The listing builds one solid part. Answer for the finished solid, in the listing's coordinates (mm). Coordinates: 2 decimals unless noted, no trailing zeros. Loops run counter-clockwise (first coordinate to the right, second up) from the corner with the lowest first, then second, coordinate; pieces in that order, holes last. Notation, with made-up numbers: (-0.75, 19) - (38.25, 19) arc R37 cw to (38.25, 58) - close; hole circle Ø3 at (27.5, 81). An arc over 180 degrees is marked (long way). Return JSON: item names as keys, results as strings. Group by question number.
1. Find the intervals of material crossed by line 1 along Z through (x, y) = (-9.25, 0.25); line 2 along Z through (x, y) = (-11, 0.35); line 3 along X through (y, z) = (0.4, 12), in increasing order.
2. Section A-A (y = 0.4) is taken. Write down the section's boundary in (x, z), and give its area (3 significant figures).
3. The mould has two halves that part along X. Classify faces 1 (the face through (-11.086, 0.493, -14.768)), 2 (the face through (0, 0.5, -16.294)), 3 (the face through (12.279, 0.507, 13.616)): pulls with the +X half, pulls with the -X half, needs draft (parallel to the pull), parting line crosses it, or undercut.
```python
from build123d import *

# Parameters (mm, degrees)
SKETCH1_W           = 25.4
SKETCH1_H           = 30.48
SKETCH1_R           = 1.5
BOSS_EXTRUDE1_DEPTH = 1
FILLET1_R           = 2
FILLET2_R           = 2
FILLET3_R           = 2
FILLET4_R           = 2


with BuildPart() as part:
    # Sketch1 → Boss-Extrude1 (new body)
    with BuildSketch(Plane(origin=(0, 0, 0), x_dir=(1, 0, 0), z_dir=(0, 1, 0))):
        with Locations((0.180037034, 1.054001786)):
            Rectangle(SKETCH1_W, SKETCH1_H)
        with Locations((-9.979962966, 13.754001786)):
            Circle(SKETCH1_R, mode=Mode.SUBTRACT)
        with Locations((-9.979962966, -11.645998214)):
            Circle(SKETCH1_R, mode=Mode.SUBTRACT)
    extrude(amount=BOSS_EXTRUDE1_DEPTH)

    # Fillet1
    fillet1_edges = [part.edges().sort_by_distance(p)[0] for p in [
        (-12.519962966, 0.5, 14.185998214),
    ]]
    fillet(fillet1_edges, radius=FILLET1_R)

    # Fillet2
    fillet2_edges = [part.edges().sort_by_distance(p)[0] for p in [
        (12.880037034, 0.5, 14.185998214),
    ]]
    fillet(fillet2_edges, radius=FILLET2_R)

    # Fillet3
    fillet3_edges = [part.edges().sort_by_distance(p)[0] for p in [
        (12.880037034, 0.5, -16.294001786),
    ]]
    fillet(fillet3_edges, radius=FILLET3_R)

    # Fillet4
    fillet4_edges = [part.edges().sort_by_distance(p)[0] for p in [
        (-12.519962966, 0.5, -16.294001786),
    ]]
    fillet(fillet4_edges, radius=FILLET4_R)


solid = part.part
```
The answers:
{
 "1": {"line 1": "z = -16.29 to -15.06, -12.44 to 10.34, 12.96 to 14.19", "line 2": "z = -16.24 to -14.85, -12.65 to 10.55, 12.75 to 14.13", "line 3": "x = -12.52 to -11.44, -8.52 to 12.88"},
 "2": {"outline": "(-12.52, -14.29) arc R2 ccw to (-10.52, -16.29) - (10.88, -16.29) arc R2 ccw to (12.88, -14.29) - (12.88, 12.19) arc R2 ccw to (10.88, 14.19) - (-10.52, 14.19) arc R2 ccw to (-12.52, 12.19) - close; hole circle Ø3 at (-9.98, -13.75); hole circle Ø3 at (-9.98, 11.65)", "area": "757 mm2"},
 "3": {"face 1": "undercut", "face 2": "needs draft", "face 3": "pulls with the +X half"}
}
